Part model, mm, in its own coordinate system. A direction names the side the tool comes from. Round coordinates to 2 decimals unless told otherwise and drop trailing zeros. Loops run counter-clockwise (first coordinate to the right, second up) from the corner with the lowest first, then second, coordinate; pieces in that order, holes last.
1) Probe line 1 (X direction, y = -4.5, z = 0.5); line 2 (Y direction, x = 4.5, z = 0.25); line 3 (Y direction, x = 43.5, z = 1.25). List the from-to ranges inside material, lowest first.
2) Drop flat-ended pins along their axis: P1, Ø0.5, axis at y = 0, z = -1.5, coming from the -X side; P2, Ø2, axis at x = 17.5, y = -2, coming from the -Z side; P3, Ø5, axis at x = 42, y = 0, coming from the -Z side. Give the stop position or say it passes through.
3) Band-saw the part on A-A, the plane y = 3.5. Write the cut outline in (x, z), then the cut area to 3 significant figures.
4) Mould opens along Y. For faces 1 (the flat face through (63.05, 0, 0)), 2 (the cylindrical face through (2.56, -1.08, -4.88)), 3 (the flat face through (2.34, 0, -1.5)), 4 (the conical face through (4.863, -0.012, 0.039)) say: +Y half, -Y half, draft (parallel to the pull), parting line (faces both ways), or undercut.
5) 3-axis set-ups, long thin cutter, end or side, ignore diameter. For faces 5 (the flat face through (2.34, -1.5, 0)), 6 (the flat face through (3.05, 2.2, -1)): which of +Z, -Z, +X, -X, +Y, -Y reach the whole face in a straight line?
6) Band-saw the part on B-B, the plane x = 50. Write the cut outline in (y, z), then the cut area to 3 significant figures.
from build123d import *

# Parameters (mm, degrees)
RECPAT_COUNT = 2
RECPAT_ANGLE = 90


with BuildPart() as part:
    # Fillet1: read off the stored shape, not the designer's step
    # Fillet1 outline → Fillet1 (revolve)
    with BuildSketch(Plane.YX):
        with BuildLine():
            Line((2, 3.25), (2, 63.05))
            Line((2, 63.05), (0, 63.05))
            Line((0, 63.05), (0, 2.05))
            Line((0, 2.05), (5, 2.05))
            Line((5, 2.05), (5, 3.05))
            Line((5, 3.05), (2.2, 3.05))
            ThreePointArc((2.2, 3.05), (2.058578644, 3.108578644), (2, 3.25))
        make_face()
    revolve(axis=Axis((0, 0, 0), (1, 0, 0)))

    # PanSke → Pan (revolve)
    with BuildSketch(Plane.XY, mode=Mode.PRIVATE) as pan_sk:
        with BuildLine():
            Line((2.05, 4.424646879), (2.05, 0))
            Line((2.05, 0), (0, 0))
            ThreePointArc((0, 0), (0.537396082, 2.438237068), (2.05, 4.424646879))
        make_face()
    revolve(pan_sk.sketch.rotate(Axis((0, 0, 0), (1, 0, 0)), 90), axis=Axis((0, 0, 0), (1, 0, 0)))

    # Sketch3 → Recess section 0
    with BuildSketch(Plane(origin=(0, 0, 0), x_dir=(0, 0, -1), z_dir=(1, 0, 0))):
        with BuildLine():
            Line((-0.515, 2.15), (0.515, 2.15))
            Line((0.515, 2.15), (0.515, -2.15))
            Line((0.515, -2.15), (-0.515, -2.15))
            Line((-0.515, -2.15), (-0.515, 2.15))
        make_face()
    # Sketch4 → Recess section 1
    with BuildSketch(Plane(origin=(2.34, 0, 0), x_dir=(0, 0, -1), z_dir=(1, 0, 0))):
        with BuildLine():
            Line((-0.515, 2.106524682), (0.515, 2.106524682))
            Line((0.515, 2.106524682), (0.515, -2.106524682))
            Line((0.515, -2.106524682), (-0.515, -2.106524682))
            Line((-0.515, -2.106524682), (-0.515, 2.106524682))
        make_face()
    recess = loft(mode=Mode.SUBTRACT)

    # RecPat: Recess ×2 about axis
    recpat_axis = Axis((0, 0, 0), (1, 0, 0))
    for i in range(1, RECPAT_COUNT):
        add(recess.rotate(recpat_axis, i * RECPAT_ANGLE / (RECPAT_COUNT - 1)), mode=Mode.SUBTRACT)

    # RecCorSke → RecessCore (revolve, cut)
    with BuildSketch(Plane.XY, mode=Mode.PRIVATE) as recesscore_sk:
        Polygon((0, 0), (0, 1.172663335), (4.6, 0.851), (4.876506661, 0), align=None)
    revolve(recesscore_sk.sketch.rotate(Axis((-3.175, 0, 0), (1, 0, 0)), 90), axis=Axis((-3.175, 0, 0), (1, 0, 0)), mode=Mode.SUBTRACT)


solid = part.part
Reported:
1. line 1: x = 2.05 to 3.05
1. line 2: y = -1.98 to -0.82, 0.82 to 1.98
1. line 3: y = -1.56 to 1.56
2. P1: stops at x = 2.34
2. P2: stops at z = -1.73
2. P3: stops at z = -2
3. outline: (2.05, -3.57) - (3.05, -3.57) - (3.05, 3.57) - (2.05, 3.57) - (2.05, 2.71) arc R4.62 ccw to (2.05, -2.71) - close
3. area: 10.4 mm2
4. face 1: draft
4. face 2: parting line
4. face 3: undercut
4. face 4: undercut
5. face 5: -X
5. face 6: +X
6. outline: circle Ø4 at (0, 0)
6. area: 12.6 mm2
